```python
from build123d import *

# Parameters (mm, degrees)
SKETCH1_W                                       = 47
SKETCH1_H                                       = 30
BOSS_STRUCTURE_DEPTH                            = 10
SKETCH2_W                                       = 70
SKETCH2_H                                       = 5
BOSS_ATTACHE_DEPTH                              = 12
SERVO_W                                         = 8
SERVO_H                                         = 4.2
SERVO_H_2                                       = 10
BOSS_SERVO_1_DEPTH                              = 12.6
BOSS_SERVO_2_DEPTH                              = 3
FILLET1_R                                       = 10
FILLET2_R                                       = 8
SKETCH4_R                                       = 1.5
CUT_EXTRUDE1_DEPTH                              = 6
CBORE_FOR_6_PAN_HEAD_MACHINE_SCREW1_D           = 4.3053
CBORE_FOR_6_PAN_HEAD_MACHINE_SCREW1_DEPTH       = 5
CBORE_FOR_6_PAN_HEAD_MACHINE_SCREW1_CBORE_D     = 11.000000098
CBORE_FOR_6_PAN_HEAD_MACHINE_SCREW1_CBORE_DEPTH = 3.000000096


with BuildPart() as part:
    # Sketch1 → Boss-Structure (new body)
    with BuildSketch(Plane(origin=(0, 0, 0), x_dir=(1, 0, 0), z_dir=(0, 1, 0))):
        Polygon((0, 35), (-10, 35), (-10, -35), (0, -35), (0, -5), align=None)
        with Locations((23.5, -20)):
            Rectangle(SKETCH1_W, SKETCH1_H)
    extrude(amount=-BOSS_STRUCTURE_DEPTH)

    # Sketch2 → Boss-Attache (add)
    with BuildSketch(Plane.ZY.offset(10)):
        with Locations((0, -2.5)):
            Rectangle(SKETCH2_W, SKETCH2_H)
    extrude(amount=BOSS_ATTACHE_DEPTH)

    # Servo → Boss-Servo_1 (add)
    with BuildSketch(Plane(origin=(0, 0, 0), x_dir=(1, 0, 0), z_dir=(0, 1, 0))):
        with Locations((11, -7.9)):
            Rectangle(SERVO_W, SERVO_H)
        with Locations((11, -17.8)):
            Rectangle(SERVO_W, SERVO_H_2)
        with Locations((43, -17.8)):
            Rectangle(SERVO_W, SERVO_H_2)
        with Locations((43, -7.9)):
            Rectangle(SERVO_W, SERVO_H)
    extrude(amount=BOSS_SERVO_1_DEPTH)

    # Sketch3<3> → Boss-Servo_2 (add)
    with BuildSketch(Plane(origin=(0, 0, 0), x_dir=(1, 0, 0), z_dir=(0, 1, 0))):
        Polygon((15, -29.3), (15, -26.3), (12, -26.3), (12, -32.3), (27, -32.3), (27, -29.3), align=None)
        Polygon((42, -26.3), (39, -26.3), (39, -29.3), (27, -29.3), (27, -32.3), (42, -32.3), align=None)
    extrude(amount=BOSS_SERVO_2_DEPTH)

    # Fillet1
    fillet1_edges = [part.edges().sort_by_distance(p)[0] for p in [
        (0, -5, -35),
    ]]
    fillet(fillet1_edges, radius=FILLET1_R)

    # Fillet2
    fillet2_edges = [part.edges().sort_by_distance(p)[0] for p in [
        (47, -5, 35),
    ]]
    fillet(fillet2_edges, radius=FILLET2_R)

    # Sketch4 → Cut-Extrude1 (cut)
    with BuildSketch(Plane(origin=(0, 12.6, 0), x_dir=(1, 0, 0), z_dir=(0, 1, 0))):
        with Locations((11, -17.8)):
            Circle(SKETCH4_R)
        with Locations((43, -17.8)):
            Circle(SKETCH4_R)
    extrude(amount=-CUT_EXTRUDE1_DEPTH, mode=Mode.SUBTRACT)

    # CBORE for #6 Pan Head Machine Screw1
    with Locations(Plane(origin=(0, 0, 0), x_dir=(1, 0, 0), z_dir=(0, 1, 0))):
        with Locations((-16, 20), (-16, -20.361423436)):
            CounterBoreHole(CBORE_FOR_6_PAN_HEAD_MACHINE_SCREW1_D / 2, CBORE_FOR_6_PAN_HEAD_MACHINE_SCREW1_CBORE_D / 2, CBORE_FOR_6_PAN_HEAD_MACHINE_SCREW1_CBORE_DEPTH, depth=CBORE_FOR_6_PAN_HEAD_MACHINE_SCREW1_DEPTH)


solid = part.part
```
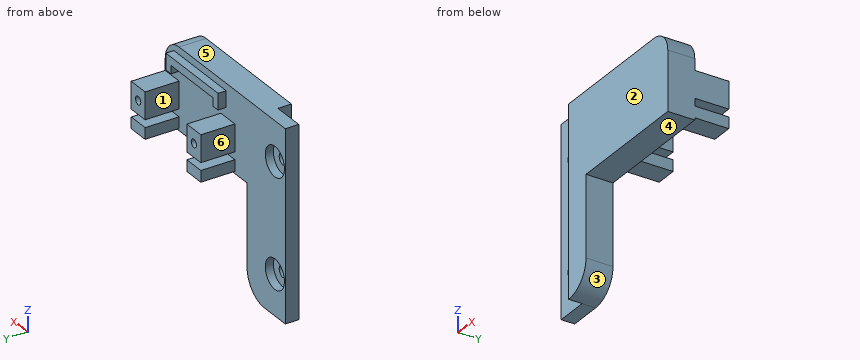
Part model, mm, in its own coordinate system. Face numbers are marked on the shaded views. A direction names the side the tool comes from. Give positions to 0.01 mm unless a question says otherwise; leave off trailing zeros. Loops run counter-clockwise (first coordinate to the right, second up) from the corner with the lowest first, then second, coordinate; pieces in that order, holes last. Notation, with made-up numbers: M 10.25,44 L 24.25,44 A11 ccw 24.25,61 Z; hole C 19,87.25 d10. An arc over 180 degrees is marked long. Return JSON: item names as keys, results as strings.
1) Saw through at B-B, the plane y = 7.75. List the corners of the cut face in (x, z), then the cut area to 3 significant figures.
Calculated:
{"outline": "M 7,5.8 L 15,5.8 L 15,10 L 7,10 Z; M 7,12.8 L 15,12.8 L 15,22.8 L 7,22.8 Z; M 39,5.8 L 47,5.8 L 47,10 L 39,10 Z; M 39,12.8 L 47,12.8 L 47,22.8 L 39,22.8 Z; hole C 11,17.8 d3; hole C 43,17.8 d3", "area": "213 mm2"}
2) Pull direction X, two halves, no side cores. Call the marked faces 1, 2 and 3: released by +X, released by -X, zero draft, split by the parting line, or undercut.
Calculated:
{"face 1": "undercut", "face 2": "zero draft", "face 3": "released by +X"}
3) Drill centre lines: line 1 (Z direction, x = -16, y = -3.9); line 2 (Z direction, x = 11, y = 9.5); line 3 (Z direction, x = 44, y = 6). Where is each one in solid material? Low to high.
Calculated:
{"line 1": "z = -35 to -22.15, -17.85 to 18.21, 22.51 to 35", "line 2": "z = 5.8 to 10, 12.8 to 16.3, 19.3 to 22.8", "line 3": "z = 5.8 to 10, 12.8 to 22.8"}
4) Saw through at C-C, the plane z = -20. List the corners of the cut face in (x, y), then the cut area to 3 significant figures.
Calculated:
{"outline": "M -22,-5 L -18.15,-5 L -18.15,-3 L -21.5,-3 L -21.5,0 L -22,0 Z; M -13.85,-5 L -10,-5 L -10,-10 L 0,-10 L 0,0 L -10.5,0 L -10.5,-3 L -13.85,-3 Z", "area": "118 mm2"}
5) Flat gauge pins, fed straight in: pin 1 Ø3.5 at (y, z) = (1, 29.5) entering from +X; pin 2 Ø0.9 at (y, z) = (1, 27) entering from +X; pin 3 Ø6.5 at (x, y) = (12, 9) entering from -Z; pin 4 Ø3.5 at (x, z) = (-16, 20.36) entering from +Y. Where does each tip first touch, or does it go through?
Calculated:
{"pin 1": "stops at x = 46.93", "pin 2": "stops at x = 42", "pin 3": "stops at z = 5.8", "pin 4": "passes through"}
6) Saw through at D-D, the plane x = 11. List the corners of the cut face in (y, z).
Calculated:
{"outline": "M -10,5 L 0,5 L 0,5.8 L 12.6,5.8 L 12.6,10 L 0,10 L 0,12.8 L 12.6,12.8 L 12.6,16.3 L 6.6,16.3 L 6.6,19.3 L 12.6,19.3 L 12.6,22.8 L 0,22.8 L 0,35 L -10,35 Z"}
7) 3-axis set-ups, long thin cutter, end or side, ignore diameter. For the marked faces 4, 5 and 6: which of +Z, -Z, +X, -X, +Y, -Y reach the whole face in a straight line?
Calculated:
{"face 4": "-Z, +X, +Y, -Y", "face 5": "+Z, +X, -X, +Y, -Y", "face 6": "+Z, -Z, -X, +Y"}
8) Saw through at A-A, the plane x = -16. List the corners of the cut face in (y, z), then the cut area to 3 significant figures.
Calculated:
{"outline": "M -5,-35 L 0,-35 L 0,-25.5 L -3,-25.5 L -3,-22.15 L -5,-22.15 Z; M -5,-17.85 L -3,-17.85 L -3,-14.5 L 0,-14.5 L 0,14.86 L -3,14.86 L -3,18.21 L -5,18.21 Z; M -5,22.51 L -3,22.51 L -3,25.86 L 0,25.86 L 0,35 L -5,35 Z", "area": "267 mm2"}
